Input: dimensioned drawing with shaded views. Units: mm. Origin: part minimum x, y, z. Give positions to 0.01 mm unless a question says otherwise; leave off trailing zeros. Order: outer loops, then holes, each group sorted by start corner. A loop starts at its lowest first (then second) coordinate and runs counter-clockwise, first axis right, second up.
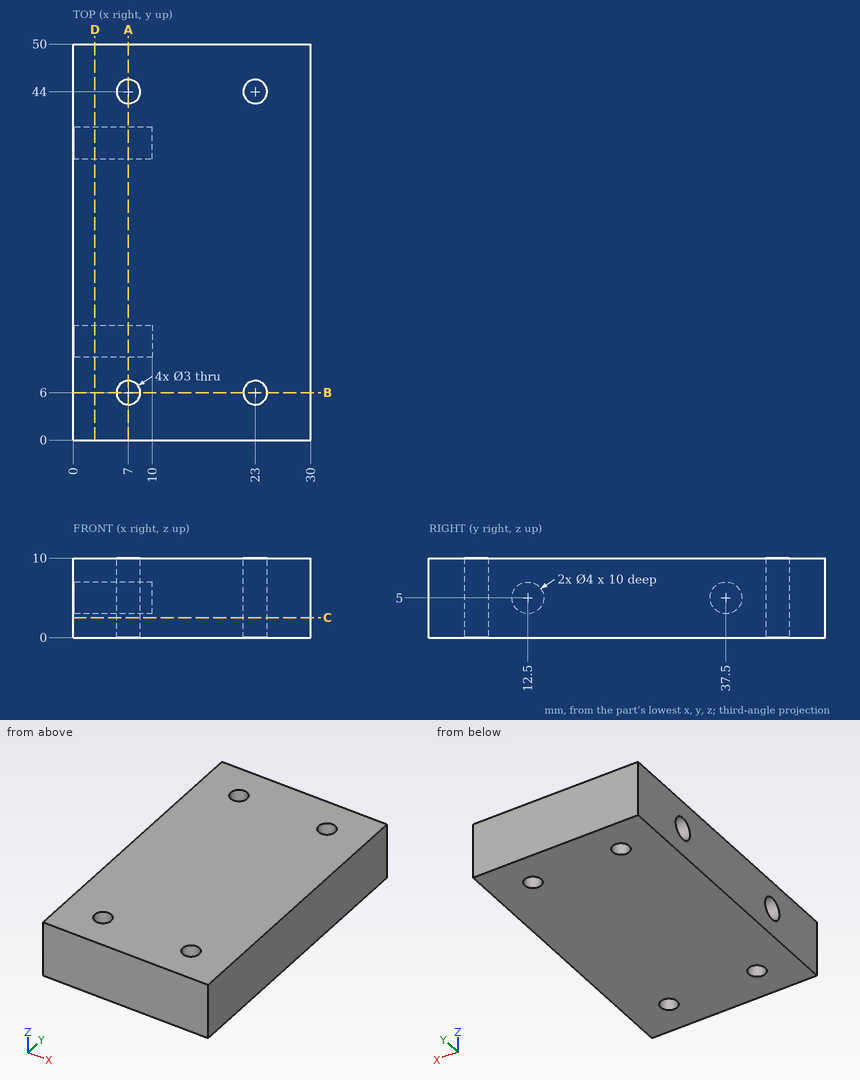
1) First-contact query: P1, Ø4, axis at x = 6, z = 3.5, coming from the -Y side; P2, Ø3, axis at y = 12.5, z = 5, coming from the -X side. Flat tips, straight axial feed; report the tip coordinate or a pass-through.
2) Line query: probe 1 along Y at (x, z) = (23, 4); probe 2 along Z at (x, y) = (2.75, 12.5); probe 3 along Y at (x, z) = (22, 2.25). Output: solid intervals per line, ascending.
3) Cut plane D-D (x = 2.75). Return the cut outline in (y, z), then the cut area to 3 significant figures.
4) Cut plane C-C (z = 2.5). Return the cut outline in (x, y), then the cut area to 3 significant figures.
5) Cut plane B-B (y = 6). Return the cut outline in (x, z).
6) Cut plane A-A (x = 7). Return the cut outline in (y, z).
Geometry says:
1. P1: stops at y = 0
1. P2: stops at x = 10
2. probe 1: y = 0 to 4.5, 7.5 to 42.5, 45.5 to 50
2. probe 2: z = 0 to 3, 7 to 10
2. probe 3: y = 0 to 4.88, 7.12 to 42.88, 45.12 to 50
3. outline: (0, 0) - (50, 0) - (50, 10) - (0, 10) - close; hole circle Ø4 at (12.5, 5); hole circle Ø4 at (37.5, 5)
3. area: 475 mm2
4. outline: (0, 0) - (30, 0) - (30, 50) - (0, 50) - close; hole circle Ø3 at (7, 6); hole circle Ø3 at (7, 44); hole circle Ø3 at (23, 6); hole circle Ø3 at (23, 44)
4. area: 1,470 mm2
5. outline: (0, 0) - (5.5, 0) - (5.5, 10) - (0, 10) - close; (8.5, 0) - (21.5, 0) - (21.5, 10) - (8.5, 10) - close; (24.5, 0) - (30, 0) - (30, 10) - (24.5, 10) - close
6. outline: (0, 0) - (4.5, 0) - (4.5, 10) - (0, 10) - close; (7.5, 0) - (42.5, 0) - (42.5, 10) - (7.5, 10) - close; (45.5, 0) - (50, 0) - (50, 10) - (45.5, 10) - close; hole circle Ø4 at (12.5, 5); hole circle Ø4 at (37.5, 5)
